Build history of the part. All positions in model axes, mm. A direction names the side the tool comes from. Give positions to 0.01 mm unless a question says otherwise; leave off trailing zeros. Loops run counter-clockwise (first coordinate to the right, second up) from the corner with the lowest first, then second, coordinate; pieces in that order, holes last. Notation, with made-up numbers: (-2, 55.25) - (48, 55.25) arc R23 cw to (48, 82.25) - close; hole circle Ø2 at (-5.75, -39). An arc over 180 degrees is marked (long way). Return JSON: item names as keys, results as strings. Group by question number.
1) Drop flat-ended pins along their axis: pin 1 (1 mm diameter, centred on x = 4.5, y = 21.5, fed in from +Z); pin 2 (5 mm diameter, centred on x = 10.5, y = -10, fed in from -Z); pin 3 (5 mm diameter, centred on x = 10, z = 15, fed in from -Y). Give the stop position or say it passes through.
2) Mould opens along X. For faces 1 (the face through (6.4, -5, -36)), 2 (the face through (11.96, -16.73, -18.24)), 3 (the face through (7, 0, 44)), 4 (the face through (11, 9, -22)) say: released by +X, released by -X, zero draft, split by the parting line, or undercut.
3) 3-axis set-ups, long thin cutter, end or side, ignore diameter. For faces 5 (the face through (12.9, 9, 22)), 6 (the face through (7, 0, -44)), 7 (the face through (10.64, 2.103, 42.677)): which of +Z, -Z, +X, -X, +Y, -Y reach the whole face in a straight line?
4) Slice it at B-B (y = 36). List the corners of the cut face in (x, z), and give its area (3 significant figures).
5) Slice it at D-D (y = 0). Count the separate pieces of the cut face and the enclosed holes in it, and give its area (3 significant figures).
6) Slice it at A-A (x = 9). List the corners of the cut face in (y, z), and give its area (3 significant figures).
7) Drill centre lines: probe 1 along Z at (x, y) = (6.75, -5.5); probe 2 along Z at (x, y) = (5, -35); probe 3 along Y at (x, z) = (10, -12.5). Where is each one in solid material? Low to high. Write a range as from..to.
```python
from build123d import *

# Parameters (mm, degrees)
DIAMETER_HOLE1_D     = 14
DIAMETER_HOLE1_DEPTH = 8.6
TAPPED_HOLE1_D       = 8.5
CUT_EXTRUDE1_DEPTH   = 65.007812023


with BuildPart() as part:
    # Sketch1 → Revolve1 (revolve)
    with BuildSketch(Plane.XY, mode=Mode.PRIVATE) as revolve1_sk:
        Polygon((15, 44), (0, 44), (0, 20.5), (2, 20.5), (2, 23.5), (11, 23.5), (11, 24.75), (12.9, 24.75), (12.9, 23.5), (15, 23.5), align=None)
    revolve(revolve1_sk.sketch.rotate(Axis((0, 0, 0), (1, 0, 0)), 90), axis=Axis((0, 0, 0), (1, 0, 0)))

    # Diameter Hole1
    with Locations(Plane(origin=(15, 0, 0), x_dir=(0, 0, -1), z_dir=(1, 0, 0))):
        with Locations((0, 36), (36, 0), (0, -36), (-36, 0)):
            Hole(DIAMETER_HOLE1_D / 2, depth=DIAMETER_HOLE1_DEPTH)

    # Tapped Hole1 (through all)
    with Locations(Plane(origin=(6.4, 0, 0), x_dir=(0, 0, -1), z_dir=(1, 0, 0))):
        with Locations((0, 36), (36, 0), (0, -36), (-36, 0)):
            Hole(TAPPED_HOLE1_D / 2)

    # Sketch6 → Cut-Extrude1 (cut, through all)
    with BuildSketch(Plane(origin=(0, 0, 0), x_dir=(0, 0, -1), z_dir=(1, 0, 0))):
        with BuildLine():
            Line((-3.516934416, 43.859219924), (-43.859219924, 3.516934416))
            ThreePointArc((-43.859219924, 3.516934416), (-31.112698372, 31.112698372), (-3.516934416, 43.859219924))
        make_face()
        with BuildLine():
            Line((3.516934416, 43.859219924), (43.859219924, 3.516934416))
            ThreePointArc((43.859219924, 3.516934416), (31.112698372, 31.112698372), (3.516934416, 43.859219924))
        make_face()
        with BuildLine():
            Line((43.859219924, -3.516934416), (3.516934416, -43.859219924))
            ThreePointArc((3.516934416, -43.859219924), (31.112698372, -31.112698372), (43.859219924, -3.516934416))
        make_face()
        with BuildLine():
            Line((-43.859219924, -3.516934416), (-3.516934416, -43.859219924))
            ThreePointArc((-3.516934416, -43.859219924), (-31.112698372, -31.112698372), (-43.859219924, -3.516934416))
        make_face()
    extrude(amount=CUT_EXTRUDE1_DEPTH, mode=Mode.SUBTRACT)


solid = part.part
```
Results:
{
 "1": {"pin 1": "z = 26.38", "pin 2": "z = -39.88", "pin 3": "y = -34.88"},
 "2": {"face 1": "released by +X", "face 2": "undercut", "face 3": "zero draft", "face 4": "undercut"},
 "3": {"face 5": "none", "face 6": "-Z, +X, -X", "face 7": "+X"},
 "4": {"outline": "(0, -11.38) - (15, -11.38) - (15, -7) - (6.4, -7) - (6.4, -4.25) - (0, -4.25) - close; (0, 4.25) - (6.4, 4.25) - (6.4, 7) - (15, 7) - (15, 11.38) - (0, 11.38) - close", "area": "166 mm2"},
 "5": {"separate pieces": "4", "enclosed holes": "0", "area": "273 mm2"},
 "6": {"outline": "(-43.86, -3.52) - (-3.52, -43.86) arc R44 ccw to (3.52, -43.86) - (43.86, -3.52) arc R44 ccw to (43.86, 3.52) - (3.52, 43.86) arc R44 ccw to (-3.52, 43.86) - (-43.86, 3.52) arc R44 ccw to start; hole circle Ø14 at (-36, 0); hole circle Ø47 at (0, 0); hole circle Ø14 at (0, -36); hole circle Ø14 at (0, 36); hole circle Ø14 at (36, 0)", "area": "2,090 mm2"},
 "7": {"probe 1": "-41.88..-40.33, -31.67..-22.85, 22.85..31.67, 40.33..41.88", "probe 2": "-12.38..-4.13, 4.13..12.38", "probe 3": "-34.88..-19.9, 19.9..34.88"}
}
